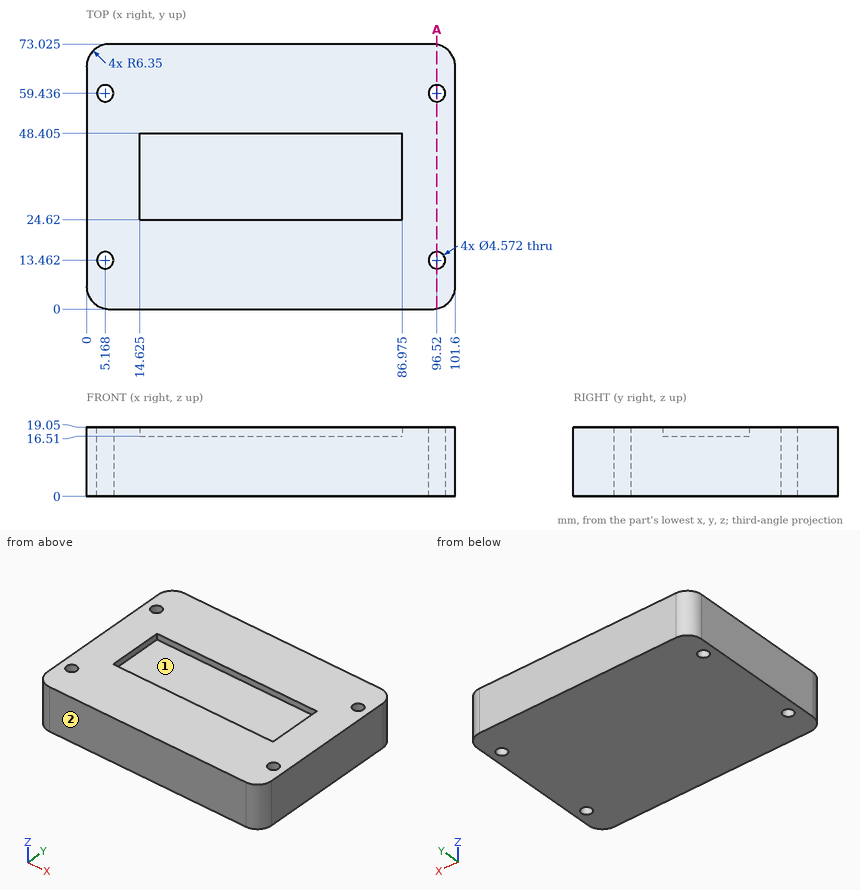
Input: dimensioned drawing with shaded views. Units: mm. Origin: part minimum x, y, z. A direction names the side the tool comes from. Round coordinates to 2 decimals unless told otherwise and drop trailing zeros. Order: outer loops, then holes, each group sorted by start corner. A loop starts at its lowest first (then second) coordinate and runs counter-clockwise, first axis right, second up. Notation, with made-up numbers: (-12, 63.5) - (41, 63.5) arc R26 cw to (41, 84.5) - close; hole circle Ø10 at (78.5, 34). An arc over 180 degrees is marked (long way). Answer as a JSON object with one key per item and string values. Group by question number.
(1) Material intervals for probe 1 along Y at (x, z) = (66.5, 17.25) (1 decimal); probe 2 along X at (y, z) = (60, 7.25) (1 decimal); probe 3 along X at (y, z) = (15, 11.5) (1 decimal), sorted ascending. Write a range as from..to.
(2) Cut plane A-A (x = 96.52). Return loops of the section in (y, z), then the cut area to 3 significant figures.
(3) Reachability of the marked faces 1 and 2 from +Z, -Z, +X, -X, +Y, -Y: full face, straight path, thin tool, end or side. Return the list, or none.
(4) Pin query (flat end, axial travel): P1, Ø3.5, axis at x = 5.17, y = 59.44, coming from the -Z side; P2, Ø7, axis at x = 62.5, y = 41.5, coming from the +Z side. Return the tip coordinate at first contact, or that it passes through.
Here are the results:
{
 "1": {"probe 1": "y = 0..24.6, 48.4..73", "probe 2": "x = 0..3, 7.4..94.3, 98.7..101.6", "probe 3": "x = 0..3.5, 6.9..94.8, 98.2..101.6"},
 "2": {"outline": "(0.13, 0) - (11.18, 0) - (11.18, 19.05) - (0.13, 19.05) - close; (15.75, 0) - (57.15, 0) - (57.15, 19.05) - (15.75, 19.05) - close; (61.72, 0) - (72.9, 0) - (72.9, 19.05) - (61.72, 19.05) - close", "area": "1,210 mm^2"},
 "3": {"face 1": "+Z", "face 2": "+Z, -Z, +X, -X, -Y"},
 "4": {"P1": "passes through", "P2": "stops at z = 16.51"}
}
